```python
from build123d import *

# Parameters (mm, degrees)
SKETCH1_R           = 14.2875
BOSS_EXTRUDE1_DEPTH = 12.7
CUT_EXTRUDE1_REACH  = 296.425
BOSS_EXTRUDE2_DEPTH = 12.7


with BuildPart() as part:
    # Sketch1 → Boss-Extrude1 (new body)
    with BuildSketch(Plane.XY):
        with BuildLine():
            ThreePointArc((15.768991732, 19.262016535), (8.527285023, 28.043059255), (-1.822173444, 32.779908077))
            ThreePointArc((-1.822173444, 32.779908077), (-39.510935789, 14.446614644), (-31.433481123, -26.678890597))
            ThreePointArc((-31.433481123, -26.678890597), (-29.629692736, -28.429204591), (-28.007722741, -30.349221507))
            Line((-28.007722741, -30.349221507), (-11.423585695, -52.076414305))
            Line((-11.423585695, -52.076414305), (25.4, -88.9))
            Line((25.4, -88.9), (69.85, -156.121724899))
            Line((69.85, -156.121724899), (76.2, -194.221724899))
            Line((76.2, -194.221724899), (101.6, -194.221724899))
            Line((101.6, -194.221724899), (107.95, -156.121724899))
            Line((107.95, -156.121724899), (152.4, -88.9))
            Line((152.4, -88.9), (189.223585695, -52.076414305))
            Line((189.223585695, -52.076414305), (205.807722741, -30.349221507))
            ThreePointArc((205.807722741, -30.349221507), (207.429692736, -28.429204591), (209.233481123, -26.678890597))
            ThreePointArc((209.233481123, -26.678890597), (217.310935789, 14.446614644), (179.622173444, 32.779908077))
            ThreePointArc((179.622173444, 32.779908077), (169.272714977, 28.043059255), (162.031008268, 19.262016535))
            Line((162.031008268, 19.262016535), (155.081549349, 5.363098697))
            ThreePointArc((155.081549349, 5.363098697), (153.948502104, 2.736916834), (153.117891795, 0))
            ThreePointArc((153.117891795, 0), (152.580111535, -2.976652205), (152.4, -5.996126628))
            Line((152.4, -5.996126628), (152.4, -14.878975516))
            ThreePointArc((152.4, -14.878975516), (150.466540126, -24.599134698), (144.960512242, -32.839487758))
            Line((144.960512242, -32.839487758), (106.860512242, -70.939487758))
            ThreePointArc((106.860512242, -70.939487758), (88.9, -78.378975516), (70.939487758, -70.939487758))
            Line((70.939487758, -70.939487758), (32.839487758, -32.839487758))
            ThreePointArc((32.839487758, -32.839487758), (27.333459874, -24.599134698), (25.4, -14.878975516))
            Line((25.4, -14.878975516), (25.4, -5.996126628))
            ThreePointArc((25.4, -5.996126628), (24.720524332, -0.160402447), (22.718450651, 5.363098697))
            Line((22.718450651, 5.363098697), (15.768991732, 19.262016535))
        make_face()
        Circle(SKETCH1_R, mode=Mode.SUBTRACT)
        with Locations((177.8, 0)):
            Circle(SKETCH1_R, mode=Mode.SUBTRACT)
    extrude(amount=BOSS_EXTRUDE1_DEPTH)

    # Sketch2 → Cut-Extrude1 (cut, up to next)
    with BuildSketch(Plane(origin=(0, 0, 0), x_dir=(-1, 0, 0), z_dir=(0, 0, -1)), mode=Mode.PRIVATE) as cut_extrude1_sk1:
        with BuildLine():
            Line((-152.4, -14.878975516), (-25.4, -14.878975516))
            ThreePointArc((-25.4, -14.878975516), (-88.9, -85.725), (-152.4, -14.878975516))
        make_face()
    cut_extrude1_tool1 = extrude(cut_extrude1_sk1.sketch, amount=-CUT_EXTRUDE1_REACH, mode=Mode.PRIVATE) & part.part
    add(cut_extrude1_tool1.solids().sort_by_distance((88.9, -45.233395, 0))[0], mode=Mode.SUBTRACT)

    # Sketch3 → Boss-Extrude2 (add, through all)
    with BuildSketch(Plane(origin=(0, 0, 0), x_dir=(-1, 0, 0), z_dir=(0, 0, -1))):
        with BuildLine():
            Line((-205.807722741, -30.349221507), (-107.95, -156.121724899))
            Line((-107.95, -156.121724899), (-69.85, -156.121724899))
            Line((-69.85, -156.121724899), (28.007722741, -30.349221507))
            Line((28.007722741, -30.349221507), (-25.01914535, -21.84414535))
            ThreePointArc((-25.01914535, -21.84414535), (-88.9, -85.725), (-152.78085465, -21.84414535))
            Line((-152.78085465, -21.84414535), (-205.807722741, -30.349221507))
        make_face()
    extrude(amount=-BOSS_EXTRUDE2_DEPTH)


solid = part.part
```
The model under review builds one solid part; all positions refer to its coordinate system, in mm. A direction names the side the tool comes from. Give positions to 0.01 mm unless a question says otherwise; leave off trailing zeros. Write each loop counter-clockwise with the first axis right and the second up, starting at its lowest first coordinate (ties: lowest second). Pieces come first, ordered by that corner, then holes. Notation, with made-up numbers: M 60.5,17 L 79.5,17 A23 ccw 79.5,41 Z; hole C 34,-22 d11. An arc over 180 degrees is marked long. Write each question's results on one line, items separated by ' | '. Start each with the question number.
1. For probe 1 along X at (y, z) = (11, 11.25); probe 2 along Y at (x, z) = (88.9, 4.75) (3 decimals); probe 3 along X at (y, z) = (-78.5, 2.5), list the stretches that pass through material, from the lowest coordinate up. Write a range as [from, to].
2. We need section C-C (x = 61). Write out the cut boundary in (y, z).
3. We need section B-B (y = -38). Write out the cut boundary in (x, z), and give its area (3 significant figures).
4. We need section D-D (y = -91). Write out the cut boundary in (x, z).
5. Insertion check: pin 1 Ø4.5 at (y, z) = (-10, 7.5) entering from +X; pin 2 Ø2 at (x, z) = (1, 5.5) entering from +Y; pin 3 Ø4 at (x, z) = (37, 3) entering from -Y; pin 4 Ø10 at (x, y) = (173.5, -13) entering from +Z. Each pin has a flat end and moves straight along its axis. Give the tip position at first contact, or say it passes through.
6. We need section A-A (z = 4.5). Count the separate pieces of the cut face and the enclosed holes in it, and give its area (3 significant figures).
7. Mouldability with a two-part tool opening along Y and no side actions: class faces 1 (the cylindrical face through (-14.274, 0.628, 6.261)), 2 (the flat face through (104.73, -175.44, 6.26)), 3 (the flat face through (25.4, -10, 6)) as released by +Y, released by -Y, zero draft, split by the parting line, or undercut.
8. For faces 4 (the flat face through (30.495, -105.54, 6.261)), 5 (the cylindrical face through (87.398, -85.707, 6.261)), 6 (the flat face through (19.3, 12.2, 6.3)), list the 3-axis set-ups (+Z, -Z, +X, -X, +Y, -Y) from which the entire face can be reached by the end or side of a thin tool; tool diameter is ignored.
Results found:
1) probe 1: x = [-41, -9.12], [9.12, 19.9], [157.9, 168.68], [186.92, 218.8] | probe 2: y = [-194.222, -85.725] | probe 3: x = [9.46, 59.39], [118.41, 168.34]
2) outline: M -144.75,0 L -79.31,0 L -79.31,12.7 L -144.75,12.7 Z
3) outline: M -22.17,0 L 27.1,0 L 27.1,12.7 L -22.17,12.7 Z; M 150.7,0 L 199.97,0 L 199.97,12.7 L 150.7,12.7 Z | area: 1,250 mm^2
4) outline: M 19.18,0 L 158.62,0 L 158.62,12.7 L 19.18,12.7 Z
5) pin 1: stops at x = 220.22 | pin 2: stops at y = 32.33 | pin 3: stops at y = -116.47 | pin 4: stops at z = 12.7
6) separate pieces: 1 | enclosed holes: 2 | area: 19,000 mm^2
7) face 1: undercut | face 2: released by -Y | face 3: zero draft
8) face 4: +Z, -Z, -X, -Y | face 5: +Z, -Z | face 6: +Z, -Z, +Y
